Print and shaded views of the part. All mm, measured from the part's lowest x, y and z. A direction names the side the tool comes from. Coordinates: 2 decimals unless noted, no trailing zeros. Loops run counter-clockwise (first coordinate to the right, second up) from the corner with the lowest first, then second, coordinate; pieces in that order, holes last.
1) Wall check: line 1 along X through (y, z) = (4, 38); line 2 along Y through (x, z) = (29, 53); line 3 along X through (y, z) = (2, 69). Give the ranges that are in metal, low to high.
2) Saw through at D-D, the plane z = 69.5. Write the cut outline in (x, y), and give its area (3 significant figures).
3) Saw through at B-B, the plane z = 38.1. Write the cut outline in (x, y), and give its area (3 significant figures).
4) Which spindle directions (+Z, -Z, +X, -X, +Y, -Y) get a long thin tool onto all of the face, cutting with end or side? Do the marked faces 1 and 2. Say none if no direction does.
5) Pin check, flat tips, straight feed: pin 1 Ø1.5 at (x, y) = (28.5, 6.5) entering from -Z; pin 2 Ø3 at (x, y) = (24, 13.5) entering from +Z; pin 3 Ø2 at (x, y) = (61.5, 5) entering from -Z. Stop position of each tip, or through.
6) Saw through at A-A, the plane x = 38.1. Write the cut outline in (y, z).
7) Saw through at C-C, the plane x = 6.35. Write the cut outline in (y, z), and give its area (3 significant figures).
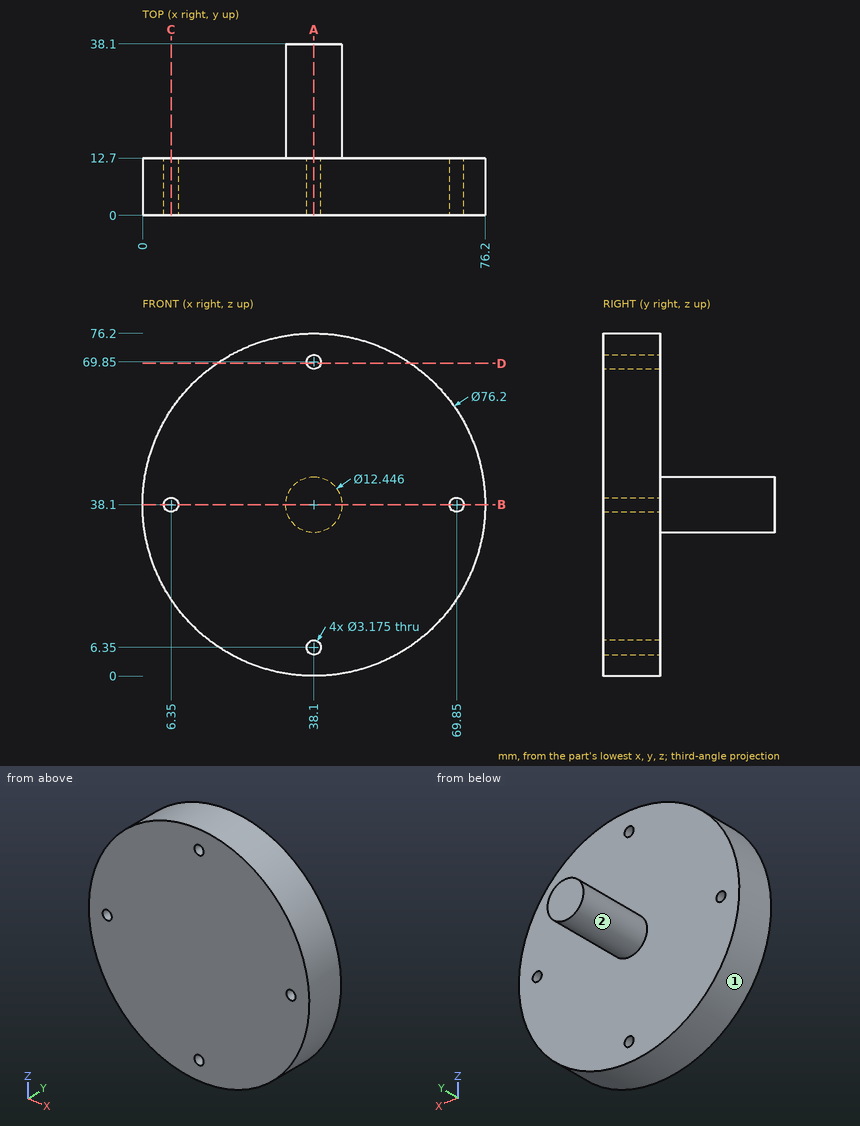
Data:
1. line 1: x = 0 to 4.77, 7.93 to 68.27, 71.43 to 76.2
1. line 2: y = 0 to 12.7
1. line 3: x = 15.81 to 36.76, 39.44 to 60.39
2. outline: (16.52, 0) - (36.55, 0) - (36.55, 12.7) - (16.52, 12.7) - close; (39.65, 0) - (59.68, 0) - (59.68, 12.7) - (39.65, 12.7) - close
2. area: 509 mm2
3. outline: (0, 0) - (4.76, 0) - (4.76, 12.7) - (0, 12.7) - close; (7.94, 0) - (68.26, 0) - (68.26, 12.7) - (44.32, 12.7) - (44.32, 38.1) - (31.88, 38.1) - (31.88, 12.7) - (7.94, 12.7) - close; (71.44, 0) - (76.2, 0) - (76.2, 12.7) - (71.44, 12.7) - close
3. area: 1,200 mm2
4. face 1: +Y, -Y
4. face 2: +Y
5. pin 1: stops at z = 1.04
5. pin 2: stops at z = 73.97
5. pin 3: stops at z = 7.28
6. outline: (0, 0) - (12.7, 0) - (12.7, 4.76) - (0, 4.76) - close; (0, 7.94) - (12.7, 7.94) - (12.7, 31.88) - (38.1, 31.88) - (38.1, 44.32) - (12.7, 44.32) - (12.7, 68.26) - (0, 68.26) - close; (0, 71.44) - (12.7, 71.44) - (12.7, 76.2) - (0, 76.2) - close
7. outline: (0, 17.04) - (12.7, 17.04) - (12.7, 36.51) - (0, 36.51) - close; (0, 39.69) - (12.7, 39.69) - (12.7, 59.16) - (0, 59.16) - close
7. area: 495 mm2
